Autodesk Inventor part; units mm, degrees
ref_plane "YZ Plane" through (0, 0, 0) normal (1, 0, 0) x (0, 1, 0)
ref_plane "XZ Plane" through (0, 0, 0) normal (0, 1, 0) x (-1, 0, 0)
ref_plane "XY Plane" through (0, 0, 0) normal (0, 0, 1) x (1, 0, 0)
sketch "Sketch1" plane through (0, 0, 0) normal (0, 1, 0) x (-1, 0, 0)
  line L0 (-13, 0) -> (3.2, 0)
  line L1 (3.2, 0) -> (3.2, 3)
  line L2 (3.2, 3) -> (-13, 3)
  line L3 (-13, 3) -> (-13, 0)
  line L4 (-13, 3) -> (-10, 3)
  line L5 (-10, 3) -> (-10, 19)
  line L6 (-10, 19) -> (-13, 19)
  line L7 (-13, 19) -> (-13, 3)
  line L8 (3.2, 3) -> (0.2, 3)
  line L9 (0.2, 3) -> (0.2, 19)
  line L10 (0.2, 19) -> (3.2, 19)
  line L11 (3.2, 19) -> (3.2, 3)
  point P0 (0, 0)
  dimension "d0" = 16.2
  dimension "d1" = 3
  dimension "d2" = 3
  dimension "d3" = 16
  dimension "d4" = 3
  dimension "d5" = 16
extrude "Extrusion1" add sketch "Sketch1" along normal blind 3
Design review of the part built by this model. Coordinates are the model's own, in mm. A direction names the side the tool comes from. Round coordinates to 2 decimals unless told otherwise and drop trailing zeros. Write each loop counter-clockwise with the first axis right and the second up, starting at its lowest first coordinate (ties: lowest second). Pieces come first, ordered by that corner, then holes. Notation, with made-up numbers: (16, 22) - (65, 22) arc R9 cw to (65, 33) - close; hole circle Ø7 at (-20.5, 54.25). An arc over 180 degrees is marked (long way). Return JSON: item names as keys, results as strings. Group by question number.
Item 1: We need section C-C on x = 3. Write out the cut boundary in (y, z).
Item 2: Insertion check: P1, Ø0.9, axis at x = 6.5, y = 1, coming from the +Z side. The pin has a flat end and moves straight along its axis. Give the tip position at first contact, or say it passes through.
Item 3: Machinability: for faces 1 (the face through (5, 1, 3)), 2 (the face through (10.4, 0, 9.6)), which of the approach directions +Z, -Z, +X, -X, +Y, -Y give a long, thin tool a straight path to every point of the face, cutting with its end or side? Answer none if there is none.
Item 4: For probe 1 along X at (y, z) = (2.05, 3.5); probe 2 along Z at (x, y) = (5, 2), list the stretches that pass through material, from the lowest coordinate up. Write a range as [from, to].
Item 5: We need section A-A on z = 5.5. Write out the cut boundary in (x, y), and give its area (3 significant figures).
Item 6: We need section B-B on y = 2.15. Write out the cut boundary in (x, z), and give its area (3 significant figures).
Model answer:
{
 "1": {"outline": "(0, 0) - (3, 0) - (3, 3) - (0, 3) - close"},
 "2": {"P1": "stops at z = 3"},
 "3": {"face 1": "+Z, +Y, -Y", "face 2": "+Z, -Z, +X, -X, -Y"},
 "4": {"probe 1": "x = [-3.2, -0.2], [10, 13]", "probe 2": "z = [0, 3]"},
 "5": {"outline": "(-3.2, 0) - (-0.2, 0) - (-0.2, 3) - (-3.2, 3) - close; (10, 0) - (13, 0) - (13, 3) - (10, 3) - close", "area": "18.0 mm²"},
 "6": {"outline": "(-3.2, 0) - (13, 0) - (13, 19) - (10, 19) - (10, 3) - (-0.2, 3) - (-0.2, 19) - (-3.2, 19) - close", "area": "145 mm²"}
}
